Here's the drawing with two shaded views (mm, measured from the low corner). I have some questions. A direction names the side the tool comes from. Round coordinates to 2 decimals unless told otherwise and drop trailing zeros. Loops run counter-clockwise (first coordinate to the right, second up) from the corner with the lowest first, then second, coordinate; pieces in that order, holes last. Notation, with made-up numbers: M 22.5,82 L 48.5,82 A28 ccw 48.5,112 Z; hole C 11,-39.75 d8. An arc over 180 degrees is marked long. Answer as a JSON object with one key per item and string values.
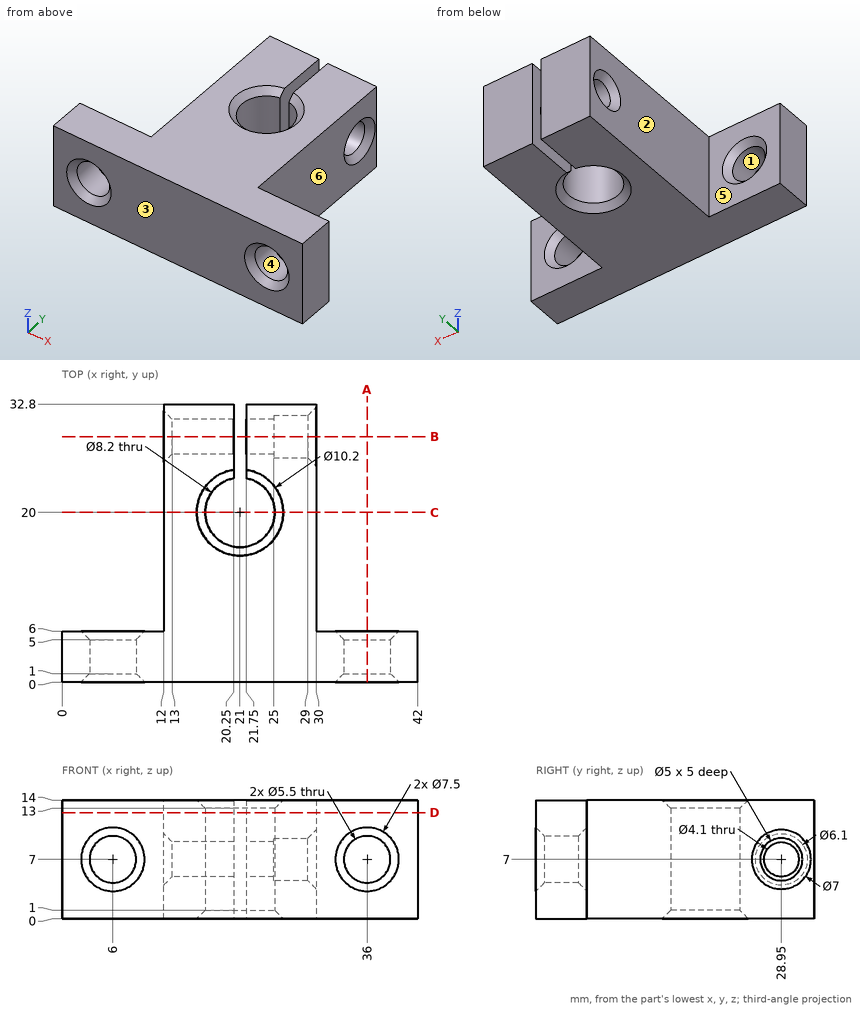
Item 1: We'd pull the mould along X, two halves only. Please class the marked faces 1, 2 and 3: +X half, -X half, draft (parallel to the pull), parting line (faces both ways), or undercut.
Solution:
{"face 1": "undercut", "face 2": "-X half", "face 3": "draft"}
Item 2: I want a section at D-D on z = 12.5. List the corners of the cut face in (x, y) for me.
Solution:
{"outline": "M 0,0 L 42,0 L 42,6 L 30,6 L 30,32.8 L 21.75,32.8 L 21.75,24.03 A4.1 cw long 20.25,24.03 L 20.25,32.8 L 12,32.8 L 12,6 L 0,6 Z"}
Item 3: I want a section at A-A on x = 36. List the corners of the cut face in (y, z) for me.
Solution:
{"outline": "M 0,0 L 6,0 L 6,3.25 L 5,4.25 L 1,4.25 L 0,3.25 Z; M 0,10.75 L 1,9.75 L 5,9.75 L 6,10.75 L 6,14 L 0,14 Z"}
Item 4: For the marked faces 4, 5 and 6, which set-ups out of +Z, -Z, +X, -X, +Y, -Y let a thin tool reach every point of the face, with its end or its side?
Solution:
{"face 4": "+Y, -Y", "face 5": "+Z, -Z, -X, +Y", "face 6": "+Z, -Z, +X, +Y"}
Item 5: I want a section at C-C on y = 20. List the corners of the cut face in (x, z) for me, plus the area to 3 significant figures.
Solution:
{"outline": "M 12,0 L 15.9,0 L 16.9,1 L 16.9,13 L 15.9,14 L 12,14 Z; M 25.1,1 L 26.1,0 L 30,0 L 30,14 L 26.1,14 L 25.1,13 Z", "area": "135 mm2"}
Item 6: If I drill on L1, parallel to X at y = 4, z = 5.5; L2, parallel to Z at x = 36, y = 3; L3, parallel to Y at x = 17.75, z = 7, over which ranges is the centre line in solid material (lowest first)? Write a range as from..to.
Solution:
{"L1": "x = 0..3.7, 8.3..33.7, 38.3..42", "L2": "z = 0..4.25, 9.75..14", "L3": "y = 0..17.5, 22.5..26.9, 31..32.8"}
Item 7: For P1, Ø6, axis at y = 16.5, z = 11.5, coming from the -X side; P2, Ø4.5, axis at y = 29.5, z = 4.5, coming from the +X side; P3, Ø6.5, axis at y = 28.95, z = 7, coming from the +X side, each with a flat end and sliding along its axis, tell me the tip position at first contact or that it passes through.
Solution:
{"P1": "stops at x = 12", "P2": "stops at x = 30", "P3": "stops at x = 29.75"}
Item 8: I want a section at B-B on y = 28.95. List the corners of the cut face in (x, z) for me, plus the area to 3 significant figures.
Solution:
{"outline": "M 12,0 L 20.25,0 L 20.25,4.95 L 13,4.95 L 12,3.95 Z; M 12,10.05 L 13,9.05 L 20.25,9.05 L 20.25,14 L 12,14 Z; M 21.75,0 L 30,0 L 30,3.5 L 29,4.5 L 25,4.5 L 25,4.95 L 21.75,4.95 Z; M 21.75,9.05 L 25,9.05 L 25,9.5 L 29,9.5 L 30,10.5 L 30,14 L 21.75,14 Z", "area": "157 mm2"}
